Autodesk Inventor part; units mm, degrees
ref_plane "YZ Plane" through (0, 0, 0) normal (1, 0, 0) x (0, 1, 0)
ref_plane "XZ Plane" through (0, 0, 0) normal (0, 1, 0) x (-1, 0, 0)
ref_plane "XY Plane" through (0, 0, 0) normal (0, 0, 1) x (1, 0, 0)
sketch "Sketch1" plane through (0, 0, 0) normal (0, 0, 1) x (1, 0, 0)
  circle A0 centre (0, 0) radius 5
  circle A1 centre (5.7, 2.25) radius 0.5
  circle A2 centre (5.7, -2.25) radius 0.5
  line L0 (0, 0) -> (12.1327, 0) construction
  arc A3 (7.2, 2.25) -> (6.3507, 3.6015) centre (5.7, 2.25) ccw
  arc A4 (6.3507, -3.6015) -> (7.2, -2.25) centre (5.7, -2.25) ccw
  line L1 (2.6029, 5.406) -> (6.3507, 3.6015)
  line L2 (2.6029, -5.406) -> (6.3507, -3.6015)
  line L3 (7.2, -2.25) -> (7.2, 2.25)
  arc A5 (2.6029, 5.406) -> (2.6029, -5.406) centre (0, 0) ccw
  dimension "d1" = 10
  dimension "d12" = 1
  dimension "d13" = 1
  dimension "d14" = 4.5
  dimension "d16" = 3
  dimension "d17" = 3
  dimension "d18" = 5.7
  dimension "d19" = 6
extrude "Extrusion1" add sketch "Sketch1" along normal mid plane 2.5
sketch "Sketch2" plane through (0, 0, 0) normal (0, 0, 1) x (1, 0, 0)
  circle A0 centre (5.7, 2.25) radius 0.5
  circle A1 centre (5.7, -2.25) radius 0.5
  line L0 (7.65, 2.25) -> (7.65, -2.25) construction
  line L1 (4.6, 2.25) -> (4.6, -2.25)
  line L2 (10.7, -2.25) -> (10.7, 2.25)
  arc A2 (10.7, 2.25) -> (4.6, 2.25) centre (7.65, 2.25) ccw
  arc A3 (4.6, -2.25) -> (10.7, -2.25) centre (7.65, -2.25) ccw
  point P0 (0, 0)
  point P1 (7.65, 0)
  dimension "d20" = 1.1
  dimension "d21" = 5
extrude "Extrusion2" cut sketch "Sketch2" along normal mid plane 1
properties part number "double spring swivel 6"
Source: CAD feature listing. Evaluate the final solid. Frame: model axes, mm. A direction names the side the tool comes from. Give positions to 0.01 mm unless a question says otherwise; leave off trailing zeros. Order: outer loops, then holes, each group sorted by start corner. A loop starts at its lowest first (then second) coordinate and runs counter-clockwise, first axis right, second up. Notation, with made-up numbers: (-12, 15.5) -> (7, 15.5) arc R28 cw to (7, 48.5) -> close; hole circle Ø4 at (-16, 10.25). An arc over 180 degrees is marked (long way). Use a Markdown table: item, result.
Q1. Material intervals for line 1 (Y direction, x = 5.7, z = -1); line 2 (X direction, y = -2, z = 0.8); line 3 (Y direction, x = 3, z = 0.7), sorted ascending. Write a range as [from, to].
A:
| item | result |
|---|---|
| line 1 | [-3.91, -2.75], [-1.75, 1.75], [2.75, 3.91] |
| line 2 | [-5.66, -4.58], [4.58, 5.27], [6.13, 7.2] |
| line 3 | [-5.21, -4], [4, 5.21] |
Q2. Access query for faces 4 (the face through (5.2, 2.23, -0.88)), 5 (the face through (4.77, -3.26, -0.01)). Directions: +Z, -Z, +X, -X, +Y, -Y. A direction counts if a zero-diameter tool reaches every point of the face in a straight line with its end or side. Return the directions, or none.
A:
| item | result |
|---|---|
| face 4 | +Z, -Z |
| face 5 | +X |
Q3. Section C-C (y = 0). Return the cut outline in (x, z).
A:
| item | result |
|---|---|
| outline | (-6, -1.25) -> (-5, -1.25) -> (-5, 1.25) -> (-6, 1.25) -> close; (5, -1.25) -> (7.2, -1.25) -> (7.2, -0.5) -> (5, -0.5) -> close; (5, 0.5) -> (7.2, 0.5) -> (7.2, 1.25) -> (5, 1.25) -> close |
Q4. Section D-D (x = 5.7). Return the cut outline in (y, z).
A:
| item | result |
|---|---|
| outline | (-3.91, -1.25) -> (-2.75, -1.25) -> (-2.75, -0.5) -> (-3.91, -0.5) -> close; (-3.91, 0.5) -> (-2.75, 0.5) -> (-2.75, 1.25) -> (-3.91, 1.25) -> close; (-1.75, -1.25) -> (1.75, -1.25) -> (1.75, -0.5) -> (-1.75, -0.5) -> close; (-1.75, 0.5) -> (1.75, 0.5) -> (1.75, 1.25) -> (-1.75, 1.25) -> close; (2.75, -1.25) -> (3.91, -1.25) -> (3.91, -0.5) -> (2.75, -0.5) -> close; (2.75, 0.5) -> (3.91, 0.5) -> (3.91, 1.25) -> (2.75, 1.25) -> close |
Q5. Section B-B (z = -0.75). Return the cut outline in (x, y).
A:
| item | result |
|---|---|
| outline | (2.6, -5.41) -> (6.35, -3.6) arc R1.5 ccw to (7.2, -2.25) -> (7.2, 2.25) arc R1.5 ccw to (6.35, 3.6) -> (2.6, 5.41) arc R6 ccw (long way) to start; hole circle Ø10 at (0, 0); hole circle Ø1 at (5.7, -2.25); hole circle Ø1 at (5.7, 2.25) |
Q6. Pull-direction query (X, two-part tool) for faces 1 (the face through (-5, 0, 0)), 2 (the face through (4.76, 3.23, -0.01)), 3 (the face through (6, 0, -0.5)); classes: +X half, -X half, draft (parallel to the pull), parting line (faces both ways), or undercut.
A:
| item | result |
|---|---|
| face 1 | undercut |
| face 2 | +X half |
| face 3 | draft |
Q7. Section A-A (x = 0). Return the cut outline in (y, z), and give its area (3 significant figures).
A:
| item | result |
|---|---|
| outline | (-6, -1.25) -> (-5, -1.25) -> (-5, 1.25) -> (-6, 1.25) -> close; (5, -1.25) -> (6, -1.25) -> (6, 1.25) -> (5, 1.25) -> close |
| area | 5.00 mm^2 |
